Part print with two shaded views. Sizes in mm from the minimum x, y, z corner. A direction names the side the tool comes from. Round coordinates to 2 decimals unless told otherwise and drop trailing zeros. Order: outer loops, then holes, each group sorted by start corner. A loop starts at its lowest first (then second) coordinate and runs counter-clockwise, first axis right, second up. Notation, with made-up numbers: (15, 61.5) - (57, 61.5) arc R14 cw to (57, 80.5) - close; hole circle Ø1 at (63, -27). An arc over 180 degrees is marked (long way). Write item = value, one per line.
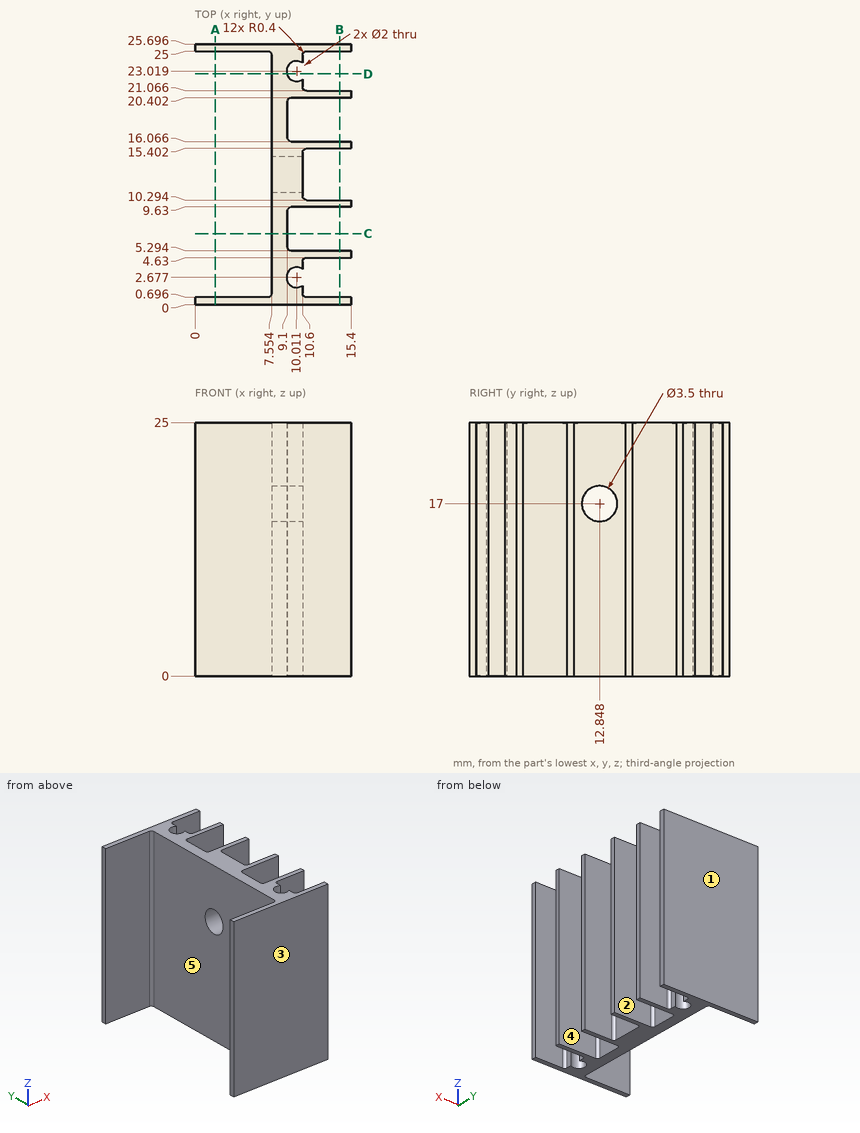
1) Cut at B-B (x = 14.25). Write the cut outline in (y, z).
Conclusion:
outline = (0, 0) - (0.7, 0) - (0.7, 25) - (0, 25) - close; (4.63, 0) - (5.29, 0) - (5.29, 25) - (4.63, 25) - close; (9.63, 0) - (10.29, 0) - (10.29, 25) - (9.63, 25) - close; (15.4, 0) - (16.07, 0) - (16.07, 25) - (15.4, 25) - close; (20.4, 0) - (21.07, 0) - (21.07, 25) - (20.4, 25) - close; (25, 0) - (25.7, 0) - (25.7, 25) - (25, 25) - close
2) Flat gauge pins, fed straight in: pin 1 Ø1.5 at (y, z) = (3, 7.5) entering from -X; pin 2 Ø0.8 at (y, z) = (1.5, 16.5) entering from +X; pin 3 Ø2 at (y, z) = (12.848, 17) entering from -X; pin 4 Ø4 at (y, z) = (7.5, 14.5) entering from +X (1 decimal). Where does each tip first touch, or does it go through?
Conclusion:
pin_1 = 7.55
pin_2 = 10.6
pin_3 = through
pin_4 = 9.2
3) Cut at A-A (x = 2). Write the cut outline in (y, z).
Conclusion:
outline = (0, 0) - (0.7, 0) - (0.7, 25) - (0, 25) - close; (25, 0) - (25.7, 0) - (25.7, 25) - (25, 25) - close
4) Cut at D-D (y = 22.75). Write the cut outline in (x, z).
Conclusion:
outline = (7.55, 0) - (9.05, 0) - (9.05, 25) - (7.55, 25) - close
5) Cut at C-C (y = 7). Write the cut outline in (x, z).
Conclusion:
outline = (7.55, 0) - (9.1, 0) - (9.1, 25) - (7.55, 25) - close
6) Mould opens along Y. For the marked faces 1, 2 and 3 say: +Y half, -Y half, draft (parallel to the pull), parting line (faces both ways), or undercut.
Conclusion:
face_1 = +Y half
face_2 = undercut
face_3 = -Y half
7) Wall check: line 1 along Y through (x, z) = (14.75, 9); line 2 along Y through (x, z) = (10, 9.25); line 3 along Y through (x, z) = (9.5, 23) (1 decimal). Give the ranges that are in metal, low to high.
Conclusion:
line_1 = 0 to 0.7, 4.63 to 5.29, 9.63 to 10.29, 15.4 to 16.07, 20.4 to 21.07, 25 to 25.7
line_2 = 0 to 1.68, 3.68 to 5.29, 9.63 to 16.07, 20.4 to 22.02, 24.02 to 25.7
line_3 = 0 to 1.8, 3.5 to 5.3, 9.6 to 16.1, 20.4 to 22.2, 23.9 to 25.7
8) 3-axis set-ups, long thin cutter, end or side, ignore diameter. For the marked faces 4 and 5: which of +Z, -Z, +X, -X, +Y, -Y reach the whole face in a straight line?
Conclusion:
face_4 = +Z, -Z, +X
face_5 = +Z, -Z, -X
